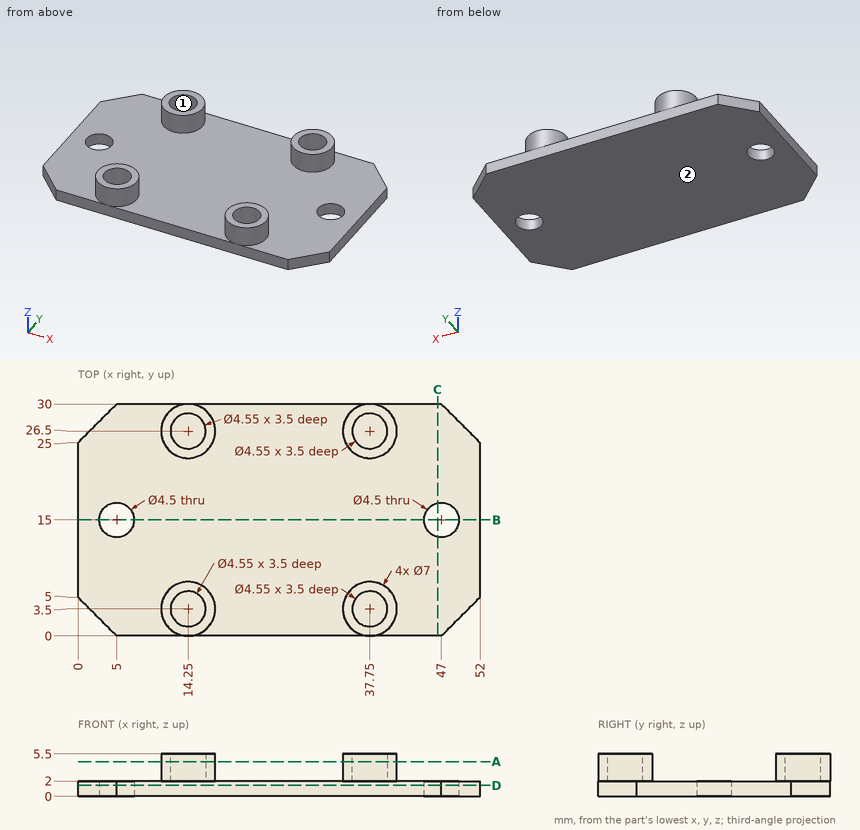
Input: dimensioned drawing with shaded views. Units: mm. Origin: part minimum x, y, z. A direction names the side the tool comes from. Coordinates: 2 decimals unless noted, no trailing zeros. Write each loop counter-clockwise with the first axis right and the second up, starting at its lowest first coordinate (ties: lowest second). Pieces come first, ordered by that corner, then holes. Notation, with made-up numbers: M 10.25,14.5 L 14.25,14.5 A15 cw 14.25,32.5 Z; hole C -24,52.5 d7. An arc over 180 degrees is marked long. Answer as a JSON object with one key per item and string values. Group by question number.
(1) Section D-D on z = 1.45. Output: boundary loops of the cut face in (x, y), plus the area to 3 significant figures.
(2) Section C-C on x = 46.5. Output: boundary loops of the cut face in (y, z).
(3) Ray query, line 1 along Y through (x, z) = (37.75, 2.9) (3 decimals); line 2 along Y through (x, z) = (15, 2.7); line 3 along Y through (x, z) = (47, 0.75). Return the intervals inside material, ascending. Write a range as [from, to].
(4) Section B-B on y = 15. Output: boundary loops of the cut face in (x, z), plus the area to 3 significant figures.
(5) Section A-A on z = 4.5. Output: boundary loops of the cut face in (x, y) (3 decimals), plus the area to 3 significant figures.
(6) Set-up query: the marked faces 1 and 2. Return all of +Z, -Z, +X, -X, +Y, -Y with unobstructed straight access to the full face (end or side cutting, diameter ignored); none if empty.
(7) Contact query for flat-ended pins moving along their axis: P1, Ø3.5, axis at x = 14.25, y = 26.5, coming from the +Z side; P2, Ø1, axis at y = 6.5, z = 3.5, coming from the +X side. Output: stop coordinate, or through.
Result set:
{
 "1": {"outline": "M 0,5 L 5,0 L 47,0 L 52,5 L 52,25 L 47,30 L 5,30 L 0,25 Z; hole C 5,15 d4.5; hole C 47,15 d4.5", "area": "1,480 mm2"},
 "2": {"outline": "M 0,0 L 12.81,0 L 12.81,2 L 0,2 Z; M 17.19,0 L 30,0 L 30,2 L 17.19,2 Z"},
 "3": {"line 1": "y = [0, 1.225], [5.775, 7], [23, 24.225], [28.775, 30]", "line 2": "y = [0.08, 1.35], [5.65, 6.92], [23.08, 24.35], [28.65, 29.92]", "line 3": "y = [0, 12.75], [17.25, 30]"},
 "4": {"outline": "M 0,0 L 2.75,0 L 2.75,2 L 0,2 Z; M 7.25,0 L 44.75,0 L 44.75,2 L 7.25,2 Z; M 49.25,0 L 52,0 L 52,2 L 49.25,2 Z", "area": "86.0 mm2"},
 "5": {"outline": "C 14.25,3.5 d7; C 14.25,26.5 d7; C 37.75,3.5 d7; C 37.75,26.5 d7; hole C 14.25,3.5 d4.55; hole C 14.25,26.5 d4.55; hole C 37.75,3.5 d4.55; hole C 37.75,26.5 d4.55", "area": "88.9 mm2"},
 "6": {"face 1": "+Z", "face 2": "-Z, +X, -X, +Y, -Y"},
 "7": {"P1": "stops at z = 2", "P2": "stops at x = 40.2"}
}
